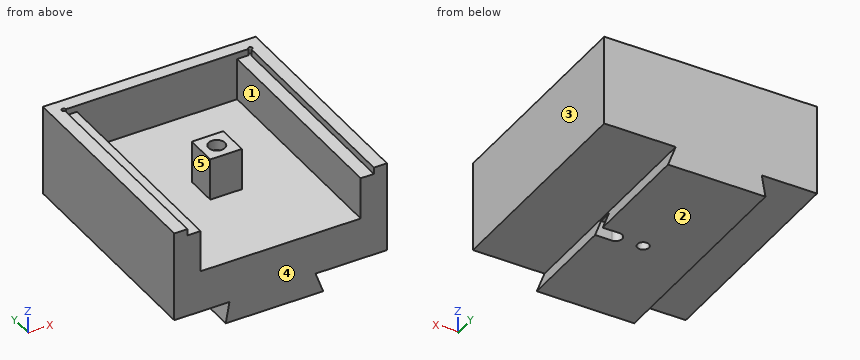
from build123d import *

# Parameters (mm, degrees)
F0_W     = 38.6842
F0_H     = 51.054
F0_W_2   = 7.62
F0_H_2   = 7.62
F0_R     = 1.9812
F0_R_2   = 1.3843
F1_DEPTH = 26.9875
F2_DEPTH = 1.5875
F3_DEPTH = 11.7475
F4_DEPTH = 4.1275
F6_DEPTH = 54.23
F8_DEPTH = 4.0386


with BuildPart() as f1:
    # F0 (on Top) → F1 (new body)
    with BuildSketch(Plane.XY):
        with Locations((0.4191, -0.127)):
            Rectangle(F0_W, F0_H)
        Rectangle(F0_W_2, F0_H_2, mode=Mode.SUBTRACT)
        with BuildLine():
            Line((26.1112, 28.575), (-25.273, 28.575))
            Line((-25.273, 28.575), (-25.273, -25.654))
            Line((-25.273, -25.654), (-22.098, -25.654))
            Line((-22.098, -25.654), (-22.098, 24.9047))
            ThreePointArc((-22.098, 24.9047), (-22.4482299887, 25.7502299887), (-21.6027, 25.4))
            Line((-21.6027, 25.4), (-18.923, 25.4))
            Line((-18.923, 25.4), (19.7612, 25.4))
            Line((19.7612, 25.4), (22.4409, 25.4))
            ThreePointArc((22.4409, 25.4), (22.9362, 25.8953), (23.4315, 25.4))
            ThreePointArc((23.4315, 25.4), (23.2864299887, 25.0497700113), (22.9362, 24.9047))
            Line((22.9362, 24.9047), (22.9362, -25.654))
            Line((22.9362, -25.654), (26.1112, -25.654))
            Line((26.1112, -25.654), (26.1112, 28.575))
        make_face()
        with BuildLine():
            Line((-22.098, 24.9047), (-22.098, -25.654))
            Line((-22.098, -25.654), (-18.923, -25.654))
            Line((-18.923, -25.654), (-18.923, 25.4))
            Line((-18.923, 25.4), (-21.6027, 25.4))
            ThreePointArc((-21.6027, 25.4), (-21.7477700113, 25.0497700113), (-22.098, 24.9047))
        make_face()
        with BuildLine():
            Line((19.7612, -25.654), (22.9362, -25.654))
            Line((22.9362, -25.654), (22.9362, 24.9047))
            ThreePointArc((22.9362, 24.9047), (22.5859700113, 25.0497700113), (22.4409, 25.4))
            Line((22.4409, 25.4), (19.7612, 25.4))
            Line((19.7612, 25.4), (19.7612, -25.654))
        make_face()
        Rectangle(F0_W_2, F0_H_2)
        Circle(F0_R, mode=Mode.SUBTRACT)
        Circle(F0_R)
        Circle(F0_R_2, mode=Mode.SUBTRACT)
        with BuildLine():
            ThreePointArc((-21.6027, 25.4), (-22.4482299887, 25.7502299887), (-22.098, 24.9047))
            Line((-22.098, 24.9047), (-22.098, 25.4))
            Line((-22.098, 25.4), (-21.6027, 25.4))
        make_face()
        with BuildLine():
            Line((22.9362, 25.4), (22.9362, 24.9047))
            ThreePointArc((22.9362, 24.9047), (23.2864299887, 25.0497700113), (23.4315, 25.4))
            ThreePointArc((23.4315, 25.4), (22.9362, 25.8953), (22.4409, 25.4))
            Line((22.4409, 25.4), (22.9362, 25.4))
        make_face()
        with BuildLine():
            Line((-22.098, 25.4), (-22.098, 24.9047))
            ThreePointArc((-22.098, 24.9047), (-21.7477700113, 25.0497700113), (-21.6027, 25.4))
            Line((-21.6027, 25.4), (-22.098, 25.4))
        make_face()
        with BuildLine():
            ThreePointArc((22.4409, 25.4), (22.5859700113, 25.0497700113), (22.9362, 24.9047))
            Line((22.9362, 24.9047), (22.9362, 25.4))
            Line((22.9362, 25.4), (22.4409, 25.4))
        make_face()
    extrude(amount=-F1_DEPTH)

    # F0 (on Top) → F2 (cut)
    with BuildSketch(Plane.XY):
        with Locations((0.4191, -0.127)):
            Rectangle(F0_W, F0_H)
        Rectangle(F0_W_2, F0_H_2, mode=Mode.SUBTRACT)
        with BuildLine():
            Line((-22.098, 24.9047), (-22.098, -25.654))
            Line((-22.098, -25.654), (-18.923, -25.654))
            Line((-18.923, -25.654), (-18.923, 25.4))
            Line((-18.923, 25.4), (-21.6027, 25.4))
            ThreePointArc((-21.6027, 25.4), (-21.7477700113, 25.0497700113), (-22.098, 24.9047))
        make_face()
        with BuildLine():
            Line((19.7612, -25.654), (22.9362, -25.654))
            Line((22.9362, -25.654), (22.9362, 24.9047))
            ThreePointArc((22.9362, 24.9047), (22.5859700113, 25.0497700113), (22.4409, 25.4))
            Line((22.4409, 25.4), (19.7612, 25.4))
            Line((19.7612, 25.4), (19.7612, -25.654))
        make_face()
        Rectangle(F0_W_2, F0_H_2)
        Circle(F0_R, mode=Mode.SUBTRACT)
        Circle(F0_R)
        Circle(F0_R_2, mode=Mode.SUBTRACT)
        with BuildLine():
            Line((22.9362, 25.4), (22.9362, 24.9047))
            ThreePointArc((22.9362, 24.9047), (23.2864299887, 25.0497700113), (23.4315, 25.4))
            ThreePointArc((23.4315, 25.4), (22.9362, 25.8953), (22.4409, 25.4))
            Line((22.4409, 25.4), (22.9362, 25.4))
        make_face()
        with BuildLine():
            ThreePointArc((-21.6027, 25.4), (-22.4482299887, 25.7502299887), (-22.098, 24.9047))
            Line((-22.098, 24.9047), (-22.098, 25.4))
            Line((-22.098, 25.4), (-21.6027, 25.4))
        make_face()
        with BuildLine():
            ThreePointArc((22.4409, 25.4), (22.5859700113, 25.0497700113), (22.9362, 24.9047))
            Line((22.9362, 24.9047), (22.9362, 25.4))
            Line((22.9362, 25.4), (22.4409, 25.4))
        make_face()
        with BuildLine():
            Line((-22.098, 25.4), (-22.098, 24.9047))
            ThreePointArc((-22.098, 24.9047), (-21.7477700113, 25.0497700113), (-21.6027, 25.4))
            Line((-21.6027, 25.4), (-22.098, 25.4))
        make_face()
    extrude(amount=-F2_DEPTH, mode=Mode.SUBTRACT)

    # F0 (on Top) → F3 (cut)
    with BuildSketch(Plane.XY):
        with Locations((0.4191, -0.127)):
            Rectangle(F0_W, F0_H)
        Rectangle(F0_W_2, F0_H_2, mode=Mode.SUBTRACT)
    extrude(amount=-F3_DEPTH, mode=Mode.SUBTRACT)

    # F0 (on Top) → F4 (cut)
    with BuildSketch(Plane.XY):
        Circle(F0_R)
        Circle(F0_R_2, mode=Mode.SUBTRACT)
    extrude(amount=-F4_DEPTH, mode=Mode.SUBTRACT)

    # F5 (on face) → F6 (cut, through all)
    with BuildSketch(Plane.XZ.offset(25.654)):
        Polygon((-11.933798938, -21.9075), (-25.273, -21.9075), (-25.273, -26.9875), (-12.82954, -26.9875), align=None)
        Polygon((26.1112, -26.9875), (26.1112, -21.9075), (8.8520512099, -21.9075), (10.70102, -26.9875), align=None)
    extrude(amount=-F6_DEPTH, mode=Mode.SUBTRACT)

    # F7 (on face) → F8 (cut)
    with BuildSketch(Plane(origin=(0, 0, -26.9875), x_dir=(1, 0, 0), z_dir=(0, 0, -1))):
        with BuildLine():
            ThreePointArc((6.6675, 1.5875), (7.7900320151, 1.1225320151), (8.255, 0))
            ThreePointArc((8.255, 0), (7.7900320151, -1.1225320151), (6.6675, -1.5875))
            Line((6.6675, -1.5875), (10.70102, -1.5875))
            Line((10.70102, -1.5875), (10.70102, 1.5875))
            Line((10.70102, 1.5875), (6.6675, 1.5875))
        make_face()
        with BuildLine():
            ThreePointArc((6.6675, -1.5875), (7.7900320151, -1.1225320151), (8.255, 0))
            ThreePointArc((8.255, 0), (7.7900320151, 1.1225320151), (6.6675, 1.5875))
            ThreePointArc((6.6675, 1.5875), (5.08, 0), (6.6675, -1.5875))
        make_face()
    extrude(amount=-F8_DEPTH, mode=Mode.SUBTRACT)


solid = f1.part
Source: CAD feature listing. Evaluate the final solid. Frame: model axes, mm. Face numbers are marked on the shaded views. A direction names the side the tool comes from. Coordinates: 2 decimals unless noted, no trailing zeros. Loops run counter-clockwise (first coordinate to the right, second up) from the corner with the lowest first, then second, coordinate; pieces in that order, holes last. Notation, with made-up numbers: (-31.75, 54) -> (-20.75, 54) arc R30 ccw to (-20.75, 85) -> close; hole circle Ø7 at (36, 48). An arc over 180 degrees is marked (long way). Answer in a Markdown table with one row per item. Add a question column.
Q1. Section D-D on y = 16.5. Return the cut outline in (x, z).
Q2. Pull-direction query (X, two-part tool) for the marked faces 3, 4 and 5; classes: pulls with the +X half, pulls with the -X half, needs draft (parallel to the pull), parting line crosses it, or undercut.
Q3. Section C-C on x = 0. Return the cut outline in (y, z) (1 decimal), and give its area (3 significant figures).
Q4. Contact query for flat-ended pins moving along their axis: pin 1 Ø2 at (x, y) = (18.5, -19.5) entering from +Z; pin 2 Ø2.5 at (x, y) = (-1, 0.5) entering from +Z; pin 3 Ø1 at (x, y) = (7, 0) entering from -Z. Output: stop coordinate, or through.
Q5. Reachability of the marked faces 1 and 2 from +Z, -Z, +X, -X, +Y, -Y: full face, straight path, thin tool, end or side. Return the list, or none.
Q6. Ray query, line 1 along Y through (x, z) = (0, -3.2) (3 decimals); line 2 along Y through (x, z) = (0, -21.25) (3 decimals); line 3 along X through (y, z) = (2.5, -10.75). Return the intervals inside material, ascending.
Q7. Section A-A on z = -7. Return the cut outline in (x, y) (3 decimals).
Computed values:
| question | item | result |
|---|---|---|
| 1 | outline | (-25.27, -21.91) -> (-11.93, -21.91) -> (-12.83, -26.99) -> (10.7, -26.99) -> (8.85, -21.91) -> (26.11, -21.91) -> (26.11, 0) -> (22.94, 0) -> (22.94, -1.59) -> (19.76, -1.59) -> (19.76, -11.75) -> (-18.92, -11.75) -> (-18.92, -1.59) -> (-22.1, -1.59) -> (-22.1, 0) -> (-25.27, 0) -> close |
| 2 | face 3 | pulls with the +X half |
| 2 | face 4 | needs draft |
| 2 | face 5 | undercut |
| 3 | outline | (-25.7, -27) -> (-1.4, -27) -> (-1.4, -4.1) -> (-2, -4.1) -> (-2, -1.6) -> (-3.8, -1.6) -> (-3.8, -11.7) -> (-25.7, -11.7) -> close; (1.4, -27) -> (28.6, -27) -> (28.6, 0) -> (25.4, 0) -> (25.4, -11.7) -> (3.8, -11.7) -> (3.8, -1.6) -> (2, -1.6) -> (2, -4.1) -> (1.4, -4.1) -> close |
| 3 | area | 868 mm^2 |
| 4 | pin 1 | stops at z = -11.75 |
| 4 | pin 2 | stops at z = -1.59 |
| 4 | pin 3 | stops at z = -22.95 |
| 5 | face 1 | +Z, -Y |
| 5 | face 2 | -Z, +X, -X, +Y, -Y |
| 6 | line 1 | y = -3.81 to -1.981, 1.981 to 3.81, 25.4 to 28.575 |
| 6 | line 2 | y = -25.654 to -1.384, 1.384 to 28.575 |
| 6 | line 3 | x = -25.27 to -18.92, -3.81 to 3.81, 19.76 to 26.11 |
| 7 | outline | (-25.273, -25.654) -> (-18.923, -25.654) -> (-18.923, 25.4) -> (19.761, 25.4) -> (19.761, -25.654) -> (26.111, -25.654) -> (26.111, 28.575) -> (-25.273, 28.575) -> close; (-3.81, -3.81) -> (3.81, -3.81) -> (3.81, 3.81) -> (-3.81, 3.81) -> close; hole circle Ø2.769 at (0, 0) |
